Input: part model. Units: mm. Frame: model coordinates. Face numbers are marked on the shaded views. Round coordinates to 2 decimals unless told otherwise and drop trailing zeros. Loops run counter-clockwise (first coordinate to the right, second up) from the corner with the lowest first, then second, coordinate; pieces in that order, holes last. Notation, with made-up numbers: (84.5, 15.5) -> (125.5, 15.5) arc R29 cw to (125.5, 51.5) -> close; hole circle Ø10 at (56, -8.5). An arc over 180 degrees is marked (long way). Answer as a JSON object with one key per item and string values. Group by question number.
Item 1: Material intervals for line 1 (X direction, y = -4, z = 0.5); line 2 (X direction, y = -2.5, z = -3.5); line 3 (Z direction, x = -4.5, y = 0), sorted ascending. Write a range as [from, to].
Item 2: Pin query (flat end, axial travel): pin 1 (0.8 mm diameter, centred on y = 0, z = 0.5, fed in from -X); pin 2 (6 mm diameter, centred on x = -4, z = 2, fed in from -Y); pin 3 (3 mm diameter, centred on x = -0.5, y = -3, fed in from -Z) (3 decimals). Return the tip coordinate at first contact, or that it passes through.
Item 3: Section query A-A on x = 16.5. Return loops of the section in (y, z) (3 decimals), and give its area (3 significant figures).
Item 4: Draft query along Z for the marked faces 1 and 2. Return one class per face: released by +Z, released by -Z, zero draft, split by the parting line, or undercut.
from build123d import *

# Parameters (mm, degrees)
DOME1_FACE_RADIUS       = 2
DOME1_HEIGHT            = 2
SKETCH2_R               = 0.5
CUT_EXTRUDE1_DEPTH      = 4
SKETCH3_R               = 0.5
SKETCH3_R_2             = 0.375
EXTRUDE_THIN1_DEPTH     = 40
SKETCH4_R               = 3.5
CUT_EXTRUDE2_DEPTH      = 6
CUT_EXTRUDE2_DEPTH_BACK = 6
SKETCH6_R               = 5
CUT_EXTRUDE3_DEPTH      = 6
CUT_EXTRUDE3_DEPTH_BACK = 6


with BuildPart() as part:
    # Sketch1 → Revolve1 (revolve)
    with BuildSketch(Plane.XY):
        with BuildLine():
            Line((0, 0), (0, 2))
            Line((0, 2), (-7.3, 3.081481481))
            Line((-7.3, 3.081481481), (-7.3, 4))
            ThreePointArc((-7.3, 4), (-7.8, 4.5), (-8.3, 4))
            Line((-8.3, 4), (-8.3, 3.22962963))
            Line((-8.3, 3.22962963), (-9.3, 3.377777778))
            Line((-9.3, 3.377777778), (-9.3, 4.2))
            ThreePointArc((-9.3, 4.2), (-9.8, 4.7), (-10.3, 4.2))
            Line((-10.3, 4.2), (-10.3, 3.525925926))
            Line((-10.3, 3.525925926), (-13.5, 4))
            Line((-13.5, 4), (-13.5, 5))
            Line((-13.5, 5), (-14, 5))
            Line((-14, 5), (-14, 3.315888293))
            Line((-14, 3.315888293), (-1, 1.389962367))
            Line((-1, 1.389962367), (-1, 0))
            Line((-1, 0), (0, 0))
        make_face()
    revolve(axis=Axis((0, 0, 0), (-1, 0, 0)))

    # Dome1: a dome of height H over a round flat face of radius A is a cap of a sphere of radius (A * A + H * H) / (2 * H)
    dome1_r = (DOME1_FACE_RADIUS * DOME1_FACE_RADIUS + DOME1_HEIGHT * DOME1_HEIGHT) / (2 * DOME1_HEIGHT)
    dome1_base = Plane((0, 0, 0), z_dir=(1, 0, 0))
    with Locations(dome1_base.offset(DOME1_HEIGHT - dome1_r)):
        dome1_ball = Sphere(dome1_r, mode=Mode.PRIVATE)
    add(split(dome1_ball, bisect_by=dome1_base, keep=Keep.TOP, mode=Mode.PRIVATE))

    # Sketch2 → Cut-Extrude1 (cut, through all)
    with BuildSketch(Plane.ZY.offset(1)):
        Circle(SKETCH2_R)
    extrude(amount=-CUT_EXTRUDE1_DEPTH, mode=Mode.SUBTRACT)

    # Sketch3 → Extrude-Thin1 (add)
    with BuildSketch(Plane.ZY.offset(1)):
        Circle(SKETCH3_R)
        Circle(SKETCH3_R_2, mode=Mode.SUBTRACT)
    extrude(amount=-EXTRUDE_THIN1_DEPTH)

    # Sketch4 → Cut-Extrude2 (cut, two sides)
    with BuildSketch(Plane(origin=(0, 0, 0), x_dir=(1, 0, 0), z_dir=(0, 1, 0))) as cut_extrude2_sk:
        with Locations((39, 3.5)):
            Circle(SKETCH4_R)
    extrude(amount=CUT_EXTRUDE2_DEPTH, mode=Mode.SUBTRACT)
    extrude(cut_extrude2_sk.sketch, amount=-CUT_EXTRUDE2_DEPTH_BACK, mode=Mode.SUBTRACT)

    # Sketch6 → Cut-Extrude3 (cut, two sides)
    with BuildSketch(Plane(origin=(0, 0, 0), x_dir=(1, 0, 0), z_dir=(0, 1, 0))) as cut_extrude3_sk:
        with Locations((41, 4.082575695)):
            Circle(SKETCH6_R)
    extrude(amount=CUT_EXTRUDE3_DEPTH, mode=Mode.SUBTRACT)
    extrude(cut_extrude3_sk.sketch, amount=-CUT_EXTRUDE3_DEPTH_BACK, mode=Mode.SUBTRACT)


solid = part.part
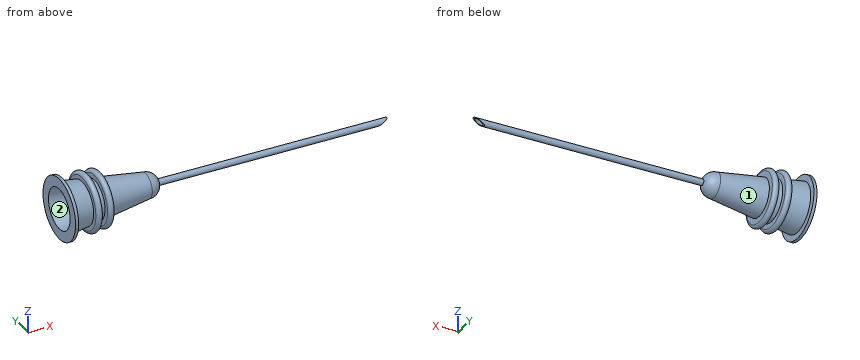
Solved:
{
 "1": {"line 1": "[-14, -13.5], [-10.3, -9.3], [-8.3, -7.3]", "line 2": "[-14, -13.5], [-10.29, -9.31], [-8.2, -7.4]", "line 3": "[-2.67, -1.91], [1.91, 2.67]"},
 "2": {"pin 1": "x = -1", "pin 2": "y = -2.94", "pin 3": "z = -1.465"},
 "3": {"outline": "circle Ø1 at (0, 0); hole circle Ø0.75 at (0, 0)", "area": "0.344 mm²"},
 "4": {"face 1": "split by the parting line", "face 2": "undercut"}
}
